from build123d import *

# Parameters (mm, degrees)
F0_R     = 49.8893389147
F1_DEPTH = 101.6
F2_W     = 30.4349269718
F2_H     = 18.0141068995
F3_DEPTH = 76.2
F4_W     = 30.4349269718
F4_H     = 76.2
F5_DEPTH = 25.4
F6_R     = 9.2441651786
F7_DEPTH = 50.8


with BuildPart() as f1:
    # F0 (on Top) → F1 (new body)
    with BuildSketch(Plane.XY):
        Circle(F0_R)
    extrude(amount=F1_DEPTH)

    # F2 (on face) → F3 (join)
    with BuildSketch(Plane.XY.offset(101.6)):
        with Locations((-15.2174634859, 9.0070534497)):
            Rectangle(F2_W, F2_H)
    extrude(amount=F3_DEPTH)

    # F4 (on face) → F5 (join)
    with BuildSketch(Plane(origin=(0, 18.0141068995, 0), x_dir=(-1, 0, 0), z_dir=(0, 1, 0))):
        with Locations((15.2174634859, 139.7)):
            Rectangle(F4_W, F4_H)
        Polygon((10.7914097607, 139.7), (17.1193554997, 157.3033481836), (24.5937909931, 139.7), align=None, mode=Mode.SUBTRACT)
    extrude(amount=F5_DEPTH)

    # F6 (on face) → F7 (cut)
    with BuildSketch(Plane.XY.offset(177.8)):
        with Locations((-12.1928649023, 21.6732509434)):
            Circle(F6_R)
    extrude(amount=-F7_DEPTH, mode=Mode.SUBTRACT)


solid = f1.part
Check sheet for the modelled part. Datum: model origin and axes. Units: mm. A direction names the side the tool comes from. Round coordinates to 2 decimals unless told otherwise and drop trailing zeros. Loops run counter-clockwise (first coordinate to the right, second up) from the corner with the lowest first, then second, coordinate; pieces in that order, holes last. Notation, with made-up numbers: M -9.75,35 L 10.25,35 A20 cw 10.25,42 Z; hole C -19.75,70 d6. An arc over 180 degrees is marked long. One line per item, written item: value.
(1) Sectioned sample at C-C, the plane x = 21. Record the cut outline in (y, z).
Computed values:
outline: M -45.25,0 L 45.25,0 L 45.25,101.6 L -45.25,101.6 Z
(2) Access from +Z, -Z, +X, -X, +Y, -Y to the whole of each face (thin tool, end or side, straight path). Record for faces 5 (the face through (-8, 43.414, 140)), 6 (the face through (-15, 0, 139)), 7 (the face through (-12, 22, 127)).
Computed values:
face 5: +Z, +X, -X, +Y
face 6: +Z, +X, -X, -Y
face 7: +Z
(3) Depth check by flat-ended pin: pin 1 Ø2 at (x, z) = (2.5, 79.5) entering from +Y; pin 2 Ø5 at (x, y) = (4, -22) entering from +Z; pin 3 Ø1 at (y, z) = (-38, 37) entering from +X. Enter the tip coordinate at first touch or a pass-through.
Computed values:
pin 1: stops at y = 49.87
pin 2: stops at z = 101.6
pin 3: stops at x = 32.9
(4) Release check for a two-part mould opening along Z. For faces 1 (the face through (-21.635, 33.359, 146.669)), 2 (the face through (-22, 21, 177.8)), 3 (the face through (-22, 18.014, 142)), 4 (the face through (-1, 1, 0)) record: +Z half, -Z half, draft (parallel to the pull), parting line (faces both ways), or undercut.
Computed values:
face 1: undercut
face 2: +Z half
face 3: undercut
face 4: -Z half
(5) Thickness scan on line 1 (Z direction, x = -4, y = -44.5); line 2 (Y direction, x = -10, z = 120); line 3 (X direction, y = 31.5, z = 155). Record the ranges inside material, lowest first.
Computed values:
line 1: z = 0 to 101.6
line 2: y = 0 to 43.41
line 3: x = -30.43 to -18.1, -16.29 to 0
(6) Sectioned sample at A-A, the plane z = 56. Record the cut outline in (x, y).
Computed values:
outline: C 0,0 d99.78
(7) Sectioned sample at B-B, the plane y = -35. Record the cut outline in (x, z), then the cut area to 3 significant figures.
Computed values:
outline: M -35.55,0 L 35.55,0 L 35.55,101.6 L -35.55,101.6 Z
area: 7,220 mm^2
